Check sheet for the modelled part. Datum: model origin and axes. Units: mm. A direction names the side the tool comes from. Give positions to 0.01 mm unless a question says otherwise; leave off trailing zeros. Write each loop counter-clockwise with the first axis right and the second up, starting at its lowest first coordinate (ties: lowest second). Pieces come first, ordered by that corner, then holes. Notation, with made-up numbers: (5, 42) -> (58, 42) arc R34 cw to (58, 81) -> close; hole circle Ø7 at (35, 45.25). An arc over 180 degrees is marked (long way). Answer as a JSON object with one key per item and string values.
from build123d import *

# Parameters (mm, degrees)
SKETCH1_R           = 16.75
BOSS_EXTRUDE1_DEPTH = 30
SKETCH2_R           = 15.2
BOSS_EXTRUDE2_DEPTH = 5
FILLET1_R           = 2
SKETCH3_R           = 15.2
BOSS_EXTRUDE3_DEPTH = 17
SKETCH4_R           = 4.95
BOSS_EXTRUDE4_DEPTH = 3.6
SKETCH5_R           = 5
BOSS_EXTRUDE5_DEPTH = 2.6
SKETCH6_R           = 1.585
BOSS_EXTRUDE6_DEPTH = 9.4
FILLET2_R           = 0.254


with BuildPart() as part:
    # Sketch1 → Boss-Extrude1 (new body)
    with BuildSketch(Plane.XY):
        Circle(SKETCH1_R)
    extrude(amount=BOSS_EXTRUDE1_DEPTH)

    # Sketch2 → Boss-Extrude2 (add)
    with BuildSketch(Plane.XY.offset(30)):
        Circle(SKETCH2_R)
    extrude(amount=BOSS_EXTRUDE2_DEPTH)

    # Fillet1
    fillet1_edges = [part.edges().sort_by_distance(p)[0] for p in [
        (-15.2, 0, 35),
    ]]
    fillet(fillet1_edges, radius=FILLET1_R)

    # Sketch3 → Boss-Extrude3 (add)
    with BuildSketch(Plane(origin=(0, 0, 0), x_dir=(-1, 0, 0), z_dir=(0, 0, -1))):
        Circle(SKETCH3_R)
    extrude(amount=BOSS_EXTRUDE3_DEPTH)

    # Sketch4 → Boss-Extrude4 (add)
    with BuildSketch(Plane.XY.offset(35)):
        Circle(SKETCH4_R)
    extrude(amount=BOSS_EXTRUDE4_DEPTH)

    # Sketch5 → Boss-Extrude5 (add)
    with BuildSketch(Plane(origin=(0, 0, -17), x_dir=(-1, 0, 0), z_dir=(0, 0, -1))):
        Circle(SKETCH5_R)
    extrude(amount=BOSS_EXTRUDE5_DEPTH)

    # Sketch6 → Boss-Extrude6 (add)
    with BuildSketch(Plane.XY.offset(38.6)):
        Circle(SKETCH6_R)
    extrude(amount=BOSS_EXTRUDE6_DEPTH)

    # Fillet2
    fillet2_edges = [part.edges().sort_by_distance(p)[0] for p in [
        (-1.585, 0, 48),
    ]]
    fillet(fillet2_edges, radius=FILLET2_R)


solid = part.part
1. Scan lines: L1, parallel to Z at x = -10, y = -5.5; L2, parallel to Z at x = 0.5, y = -3; L3, parallel to Y at x = 0.5, z = 33.5. Record each from-to range of solid material in increasing order. Write a range as [from, to].
Determined:
{"L1": "[-17, 35]", "L2": "[-19.6, 38.6]", "L3": "[-15.13, 15.13]"}
2. Sectioned sample at C-C, the plane z = 28. Enter the section's corners in (x, y).
Determined:
{"outline": "circle Ø33.5 at (0, 0)"}
3. Sectioned sample at A-A, the plane x = 0. Enter the section's corners in (y, z) (3 decimals).
Determined:
{"outline": "(-16.75, 0) -> (-15.2, 0) -> (-15.2, -17) -> (-5, -17) -> (-5, -19.6) -> (5, -19.6) -> (5, -17) -> (15.2, -17) -> (15.2, 0) -> (16.75, 0) -> (16.75, 30) -> (15.2, 30) -> (15.2, 33) arc R2 ccw to (13.2, 35) -> (4.95, 35) -> (4.95, 38.6) -> (1.585, 38.6) -> (1.585, 47.746) arc R0.254 ccw to (1.331, 48) -> (-1.331, 48) arc R0.254 ccw to (-1.585, 47.746) -> (-1.585, 38.6) -> (-4.95, 38.6) -> (-4.95, 35) -> (-13.2, 35) arc R2 ccw to (-15.2, 33) -> (-15.2, 30) -> (-16.75, 30) -> close"}
4. Go/stop test with flat-tipped pins: P1, Ø8, axis at y = -6.5, z = 10.5, coming from the -X side; P2, Ø12, axis at y = -8.5, z = 36, coming from the +X side; P3, Ø5, axis at y = -10, z = -11, coming from the +X side. Record where each tip stops, or that it passes through.
Determined:
{"P1": "x = -16.56", "P2": "x = 14.85", "P3": "x = 13.22"}
5. Mould release check, pull along Y, two halves, no side actions. Record for faces 4 (the face through (-3.63, -16.35, 14.79)), 5 (the face through (0, 0, 48)): released by +Y, released by -Y, zero draft, split by the parting line, or undercut.
Determined:
{"face 4": "split by the parting line", "face 5": "zero draft"}
6. Access from +Z, -Z, +X, -X, +Y, -Y to the whole of each face (thin tool, end or side, straight path). Record for faces 1 (the face through (4, -15, 30)), 2 (the face through (4, -15, 0)), 3 (the face through (0, 0, -19.6)).
Determined:
{"face 1": "+Z", "face 2": "-Z", "face 3": "-Z, +X, -X, +Y, -Y"}
